For this review, take the finished solid that the model builds, in its own axes (mm). Coordinates: 2 decimals unless noted, no trailing zeros. Loops run counter-clockwise (first coordinate to the right, second up) from the corner with the lowest first, then second, coordinate; pieces in that order, holes last.
1. Take a section at A-A, the plane z = 14.5. State the section outline as (x, y) points.
2. To check wall thickness, follow probe 1 along Y at (x, z) = (3.05, 14.5); probe 2 along Z at (x, y) = (5.75, 2); probe 3 along Y at (x, z) = (0.75, 116). State the ranges of each line that lie inside material, in increasing order.
3. Take a section at B-B, the plane x = 4. State the section outline as (y, z) points.
4. Clearance check with flat-ended pins moving along their axes: P1, Ø12, axis at y = 15.5, z = 16, coming from the -X side; P2, Ø5, axis at y = 12.5, z = 109.5, coming from the +X side; P3, Ø1.5, axis at x = 4, y = 12, coming from the +Z side; P4, Ø1.5, axis at x = 5, y = 12, coming from the -Z side. State where each tip first meets the part, or that it passes through.
Autodesk Inventor part; units mm, degrees
ref_plane "YZ Plane" through (0, 0, 0) normal (1, 0, 0) x (0, 1, 0)
ref_plane "XZ Plane" through (0, 0, 0) normal (0, 1, 0) x (-1, 0, 0)
ref_plane "XY Plane" through (0, 0, 0) normal (0, 0, 1) x (1, 0, 0)
sketch "Skizze1" plane through (0, 0, 0) normal (1, 0, 0) x (0, 1, 0)
  line L0 (0, 0) -> (25, 0)
  line L1 (25, 0) -> (25, 124)
  line L2 (25, 124) -> (0, 124)
  line L3 (0, 124) -> (0, 0)
  dimension "d0" = 25
  dimension "d1" = 124
extrude "Extrusion1" add sketch "Skizze1" along normal blind 8
fillet "Rundung1" radius 5 4 edges at (4, 25, 124) (4, 0, 124) (4, 25, 0) (4, 0, 0)
sketch "Skizze2" plane through (8, 0, 0) normal (1, 0, 0) x (0, 0, -1)
  circle A0 centre (-14.5, 12.5) radius 2.25
  circle A1 centre (-109.5, 12.5) radius 2.25
  line L0 (-124, 20) -> (-124, 5)
  line L1 (-5, 25) -> (-119, 25)
  point P0 (0, 0)
  dimension "d5" = 4.5
  dimension "d6" = 4.5
  dimension "d7" = 95
  dimension "d8" = 14.5
  dimension "d9" = 12.5
  dimension "d10" = 12.5
extrude "Extrusion2" cut sketch "Skizze2" against normal through all
sketch "Skizze3" plane through (0, 5, 0) normal (0, 0, -1) x (-1, 0, 0)
  circle A0 centre (-4, 7.5) radius 2.5
  line L0 (0, 20) -> (-8, 20)
  line L1 (-8, 0) -> (-8, 15)
  point P0 (0, -5)
  point P1 (-4, 20)
  dimension "d14" = 5
  dimension "d15" = 12.5
  dimension "d16" = 4
extrude "Extrusion3" cut sketch "Skizze3" against normal blind 10
sketch "Skizze4" plane through (0, 5, 124) normal (0, 0, 1) x (1, 0, 0)
  circle A0 centre (4, 7.5) radius 2.5
  point P0 (0, -5)
extrude "Extrusion4" cut sketch "Skizze4" against normal blind 10
chamfer "Fase1" distance 1 angle 45 2 edges at (1.5, 12.5, 124) (6.5, 12.5, 0)
fillet "Rundung3" radius 1 16 edges at (8, 23.5355, 1.4645) (8, 25, 62) (8, 23.5355, 122.5355) (8, 12.5, 124) (8, 1.4645, 122.5355) (8, 0, 62) (8, 1.4645, 1.4645) (8, 12.5, 0) (0, 23.5355, 1.4645) (0, 25, 62) (0, 23.5355, 122.5355) (0, 12.5, 124) (0, 1.4645, 122.5355) (0, 0, 62) (0, 1.4645, 1.4645) (0, 12.5, 0)
chamfer "Fase2" distance 1 angle 45 4 edges at (8, 12.5, 111.75) (8, 12.5, 16.75) (0, 12.5, 16.75) (0, 12.5, 111.75)
properties part number "Camera_Adapter"
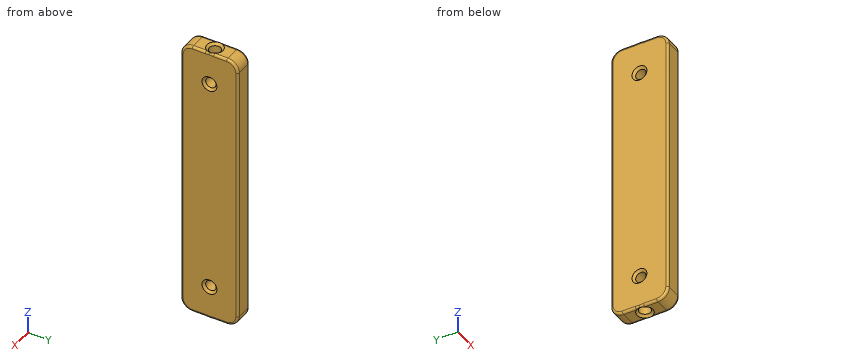
Results list:
1. outline: (0, 1) arc R1 ccw to (1, 0) - (7, 0) arc R1 ccw to (8, 1) - (8, 9.25) - (7, 10.25) - (1, 10.25) - (0, 9.25) - close; (0, 15.75) - (1, 14.75) - (7, 14.75) - (8, 15.75) - (8, 24) arc R1 ccw to (7, 25) - (1, 25) arc R1 ccw to (0, 24) - close
2. probe 1: y = 0 to 10.25, 14.75 to 25
2. probe 2: z = 1 to 123
2. probe 3: y = 0.03 to 24.97
3. outline: (0, 5) arc R5 ccw to (5, 0) - (9, 0) - (10, 1) - (10, 10) - (15, 10) - (15, 1) - (16, 0) - (20, 0) arc R5 ccw to (25, 5) - (25, 119) arc R5 ccw to (20, 124) - (16, 124) - (15, 123) - (15, 114) - (10, 114) - (10, 123) - (9, 124) - (5, 124) arc R5 ccw to (0, 119) - close; hole circle Ø4.5 at (12.5, 14.5); hole circle Ø4.5 at (12.5, 109.5)
4. P1: stops at x = 0
4. P2: stops at x = 7.25
4. P3: stops at z = 114
4. P4: stops at z = 10
